The listing builds one solid part. Answer for the finished solid, in the listing's coordinates (mm). A direction names the side the tool comes from. Coordinates: 2 decimals unless noted, no trailing zeros. Order: outer loops, then holes, each group sorted by start corner. A loop starts at its lowest first (then second) coordinate and runs counter-clockwise, first axis right, second up.
from build123d import *

# Parameters (mm, degrees)
SKICA1_R                 = 5.25
P_IDAT_VYSUNUT_M1_DEPTH  = 6
SKICA2_R                 = 11
P_IDAT_VYSUNUT_M2_DEPTH  = 5
SKICA3_W                 = 36.875028654
SKICA3_H                 = 156.768575318
SKICA3_W_2               = 39.825030946
SKICA3_H_2               = 162.668579902
ODEBRAT_VYSUNUT_M1_DEPTH = 10
ZAOBLIT1_R               = 5
SKICA4_R                 = 5
P_IDAT_VYSUNUT_M3_DEPTH  = 50


with BuildPart() as part:
    # Skica1 → Přidat vysunutím1 (new body)
    with BuildSketch(Plane.XY):
        with BuildLine():
            Line((-17.5, -62.310889132), (-17.5, 62.310889132))
            ThreePointArc((-17.5, 62.310889132), (0, 67), (17.5, 62.310889132))
            Line((17.5, 62.310889132), (17.5, -62.310889132))
            ThreePointArc((17.5, -62.310889132), (0, -67), (-17.5, -62.310889132))
        make_face()
        with Locations((0, 52)):
            Circle(SKICA1_R, mode=Mode.SUBTRACT)
        with Locations((0, 32)):
            Circle(SKICA1_R, mode=Mode.SUBTRACT)
    extrude(amount=P_IDAT_VYSUNUT_M1_DEPTH)

    # Skica2 → Přidat vysunutím2 (add)
    with BuildSketch(Plane.XY.offset(6)):
        with Locations((0, -48)):
            Circle(SKICA2_R)
    extrude(amount=P_IDAT_VYSUNUT_M2_DEPTH)

    # Skica3 → Odebrat vysunutím1 (cut)
    with BuildSketch(Plane.XY.offset(6)):
        with Locations((33.437514327, 0)):
            Rectangle(SKICA3_W, SKICA3_H)
        with Locations((-34.912515473, 0)):
            Rectangle(SKICA3_W_2, SKICA3_H_2)
    extrude(amount=-ODEBRAT_VYSUNUT_M1_DEPTH, mode=Mode.SUBTRACT)

    # Zaoblit1
    zaoblit1_edges = [part.edges().sort_by_distance(p)[0] for p in [
        (-11, -48, 6),
    ]]
    fillet(zaoblit1_edges, radius=ZAOBLIT1_R - 0.0001)  # a hair under: the kernel refuses the full size

    # Skica4 → Přidat vysunutím3 (add)
    with BuildSketch(Plane.XY.offset(11)):
        with Locations((0, -48)):
            Circle(SKICA4_R)
    extrude(amount=P_IDAT_VYSUNUT_M3_DEPTH)


solid = part.part
1) Determine the mould class of faces 1 (the face through (0, 67, 3)), 2 (the face through (0, -48, 61)), 3 (the face through (-0.683, 37.205, 2.958)) for opening direction Y: released by +Y, released by -Y, zero draft, split by the parting line, or undercut.
2) Section B-B (x = 0) is taken. Give the number of separate pieces and of enclosed holes in the cut face, then the cut area to 3 significant figures.
3) Section D-D (y = 54) is taken. Give the vertices of the cut face in (x, z), then the cut area to 3 significant figures.
4) Section A-A (y = 32) is taken. Give the vertices of the cut face in (x, z).
5) A tool of negligible diameter and unlimited length cuts with its end or side. For faces 4 (the face through (2, -53, 11)), 5 (the face through (0.1, -64.2, 6)), 6 (the face through (15, -1, 3)), from which of +Z, -Z, +X, -X, +Y, -Y can it reach the whole face along a straight path? Write none if from no direction.
6) Consider L1, parallel to Z at x = 2, y = 22.5; L2, parallel to Y at x = -1.5, z = 3.5; L3, parallel to Z at x = -1, y = -56.5. Determine where each line is inside the solid, lowest interval first.
7) Section C-C (z = 39.5) is taken. Give the vertices of the cut face in (x, y).
8) Each of these flat-tipped pins is pushed along its axis until it touches: P1, Ø6, axis at x = -10.5, z = 16.5, coming from the +Y side; P2, Ø12, axis at y = -42, z = 26, coming from the +X side; P3, Ø10, axis at x = -9, y = 31, coming from the +Z side; P4, Ø4, axis at x = -5.5, y = -61.5, coming from the +Z side (3 decimals). Where does it stop, or does it pass through?
Filled sheet:
1. face 1: released by +Y
1. face 2: zero draft
1. face 3: undercut
2. separate pieces: 3
2. enclosed holes: 0
2. area: 1,300 mm2
3. outline: (-15, 0) - (-4.85, 0) - (-4.85, 6) - (-15, 6) - close; (4.85, 0) - (15, 0) - (15, 6) - (4.85, 6) - close
3. area: 122 mm2
4. outline: (-15, 0) - (-5.25, 0) - (-5.25, 6) - (-15, 6) - close; (5.25, 0) - (15, 0) - (15, 6) - (5.25, 6) - close
5. face 4: +Z
5. face 5: +Z, -Y
5. face 6: +Z, -Z, +X, +Y, -Y
6. L1: z = 0 to 6
6. L2: y = -66.97 to 26.97, 37.03 to 46.97, 57.03 to 66.97
6. L3: z = 0 to 11
7. outline: circle Ø10 at (0, -48)
8. P1: passes through
8. P2: stops at x = 5
8. P3: stops at z = 6
8. P4: stops at z = 7.355
